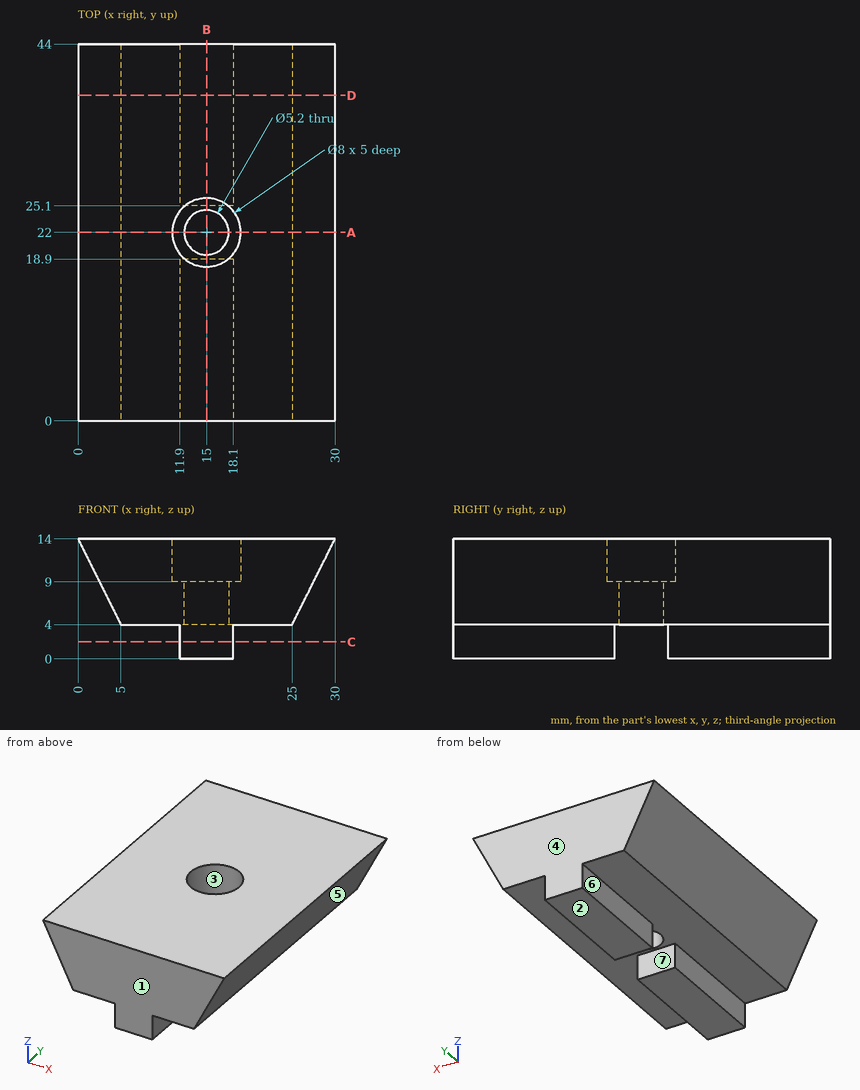
Geometry check sheet. Reference: drawing and pictorial views, mm from the part's lowest x, y, z. A direction names the side the tool comes from. Round coordinates to 2 decimals unless told otherwise and drop trailing zeros. Order: outer loops, then holes, each group sorted by start corner. A loop starts at its lowest first (then second) coordinate and runs counter-clockwise, first axis right, second up. Notation, with made-up numbers: (19.5, 84.5) -> (66.5, 84.5) arc R5 cw to (66.5, 91.5) -> close; hole circle Ø4 at (23.25, 19). An arc over 180 degrees is marked (long way). One line per item, written item: value. Start each with the question number.
Q1. Thickness scan on line 1 (Y direction, x = 15, z = 6.4); line 2 (Z direction, x = 23.5, y = 14); line 3 (X direction, y = 15.5, z = 2.5). Record the ranges inside material, lowest first.
Q2. Set-up check for the marked faces 5, 6 and 7: record each of +Z, -Z, +X, -X, +Y, -Y from which the full face is reachable in a straight line by a thin tool's end or side.
Q3. Cross-section at D-D (y = 38). Record the boundary of the cut face in (x, z), and give its area (3 significant figures).
Q4. Cross-section at B-B (x = 15). Record the boundary of the cut face in (y, z), and give its area (3 significant figures).
Q5. Cross-section at C-C (z = 2). Record the boundary of the cut face in (x, y).
Q6. Gauge pin test, flat ends, axial feed: pin 1 Ø1.2 at (y, z) = (31.5, 1.5) entering from +X; pin 2 Ø1.5 at (y, z) = (14, 8.5) entering from -X (3 decimals); pin 3 Ø1 at (x, y) = (17.5, 22) entering from -Z. Record the tip position at first contact, or that the pin passes through.
Q7. Mould release check, pull along Y, two halves, no side actions. Record for the marked faces 1, 2, 3 and 4: pulls with the +Y half, pulls with the -Y half, needs draft (parallel to the pull), parting line crosses it, or undercut.
Q8. Cross-section at A-A (y = 22). Record the boundary of the cut face in (x, z), and give its area (3 significant figures).
Completed:
1. line 1: y = 0 to 19.4, 24.6 to 44
1. line 2: z = 4 to 14
1. line 3: x = 11.9 to 18.1
2. face 5: -Z, +X, +Y, -Y
2. face 6: -Z, -X, +Y, -Y
2. face 7: -Z, +X, -X
3. outline: (0, 14) -> (5, 4) -> (11.9, 4) -> (11.9, 0) -> (18.1, 0) -> (18.1, 4) -> (25, 4) -> (30, 14) -> close
3. area: 275 mm²
4. outline: (0, 0) -> (18.9, 0) -> (18.9, 4) -> (19.4, 4) -> (19.4, 9) -> (18, 9) -> (18, 14) -> (0, 14) -> close; (24.6, 4) -> (25.1, 4) -> (25.1, 0) -> (44, 0) -> (44, 14) -> (26, 14) -> (26, 9) -> (24.6, 9) -> close
4. area: 525 mm²
5. outline: (11.9, 0) -> (18.1, 0) -> (18.1, 18.9) -> (11.9, 18.9) -> close; (11.9, 25.1) -> (18.1, 25.1) -> (18.1, 44) -> (11.9, 44) -> close
6. pin 1: stops at x = 18.1
6. pin 2: stops at x = 2.375
6. pin 3: stops at z = 4
7. face 1: pulls with the -Y half
7. face 2: needs draft
7. face 3: undercut
7. face 4: pulls with the +Y half
8. outline: (0, 14) -> (5, 4) -> (12.4, 4) -> (12.4, 9) -> (11, 9) -> (11, 14) -> close; (17.6, 4) -> (25, 4) -> (30, 14) -> (19, 14) -> (19, 9) -> (17.6, 9) -> close
8. area: 184 mm²
